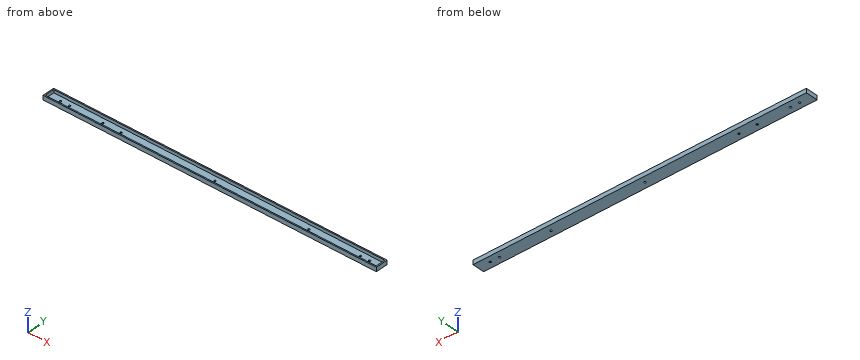
from build123d import *

# Parameters (mm, degrees)
SKETCH_1_W          = 550
SKETCH_1_H          = 20
EXTRUDE_1_DEPTH     = 7
SKETCH_2_W          = 546
SKETCH_2_H          = 16
CUT_EXTRUDE_1_DEPTH = 5
SKETCH_3_R          = 1.6
CUT_EXTRUDE_2_DEPTH = 276.270775783
SKETCH_4_R          = 1.6
CUT_EXTRUDE_3_DEPTH = 276.270775783


with BuildPart() as part:
    # ｽｹｯﾁ1 → ﾎﾞｽ - 押し出し1 (new body)
    with BuildSketch(Plane.XY):
        Rectangle(SKETCH_1_W, SKETCH_1_H)
    extrude(amount=EXTRUDE_1_DEPTH)

    # ｽｹｯﾁ2 → ｶｯﾄ - 押し出し1 (cut)
    with BuildSketch(Plane.XY.offset(7)):
        Rectangle(SKETCH_2_W, SKETCH_2_H)
    extrude(amount=-CUT_EXTRUDE_1_DEPTH, mode=Mode.SUBTRACT)

    # ｽｹｯﾁ3 → ｶｯﾄ - 押し出し2 (cut, through all)
    with BuildSketch(Plane(origin=(0, 0, 0), x_dir=(-1, 0, 0), z_dir=(0, 0, -1))):
        with Locations((255, 0)):
            Circle(SKETCH_3_R)
        with Locations((240, 0)):
            Circle(SKETCH_3_R)
        with Locations((155, 0)):
            Circle(SKETCH_3_R)
        Circle(SKETCH_3_R)
        with Locations(Location((-255, 0, 0), (0, 0, 180))):
            Circle(SKETCH_3_R)
        with Locations(Location((-240, 0, 0), (0, 0, 180))):
            Circle(SKETCH_3_R)
        with Locations(Location((-155, 0, 0), (0, 0, 180))):
            Circle(SKETCH_3_R)
    extrude(amount=-CUT_EXTRUDE_2_DEPTH, mode=Mode.SUBTRACT)

    # ｽｹｯﾁ4 → ｶｯﾄ - 押し出し3 (cut, through all)
    with BuildSketch(Plane(origin=(0, 0, 0), x_dir=(-1, 0, 0), z_dir=(0, 0, -1))):
        with Locations((185, 0)):
            Circle(SKETCH_4_R)
    extrude(amount=-CUT_EXTRUDE_3_DEPTH, mode=Mode.SUBTRACT)


solid = part.part
The model under review builds one solid part; all positions refer to its coordinate system, in mm. Coordinates: 2 decimals unless noted, no trailing zeros. Loops run counter-clockwise (first coordinate to the right, second up) from the corner with the lowest first, then second, coordinate; pieces in that order, holes last. Notation, with made-up numbers: (17, 76.25) -> (64, 76.25) arc R22 ccw to (64, 108.25) -> close; hole circle Ø4 at (-35.75, 0). An arc over 180 degrees is marked (long way). Use a Markdown table: item, result. Add a question column.
1. Clearance check with flat-ended pins moving along their axes: pin 1 Ø3.5 at (x, y) = (-155, 0) entering from -Z; pin 2 Ø3 at (x, y) = (255, 0) entering from -Z; pin 3 Ø5 at (x, y) = (68.5, 0.5) entering from +Z. State where each tip first meets the part, or that it passes through.
2. Add section A-A on z = 3.75. Write out the cut boundary in (x, y), plus the area to 3 significant figures.
3. To check wall thickness, follow line 1 (X direction, y = -2.5, z = 6); line 2 (Y direction, x = 7, z = 4.5); line 3 (Y direction, x = 0, z = 0.8). State the ranges of each line that lie inside material, in increasing order.
4. Add section B-B on x = 114.5. Write out the cut boundary in (y, z), plus the area to 3 significant figures.
Returned:
| question | item | result |
|---|---|---|
| 1 | pin 1 | stops at z = 0 |
| 1 | pin 2 | passes through |
| 1 | pin 3 | stops at z = 2 |
| 2 | outline | (-275, -10) -> (275, -10) -> (275, 10) -> (-275, 10) -> close; hole (-273, -8) -> (273, -8) -> (273, 8) -> (-273, 8) -> close |
| 2 | area | 2,260 mm² |
| 3 | line 1 | x = -275 to -273, 273 to 275 |
| 3 | line 2 | y = -10 to -8, 8 to 10 |
| 3 | line 3 | y = -10 to -1.6, 1.6 to 10 |
| 4 | outline | (-10, 0) -> (10, 0) -> (10, 7) -> (8, 7) -> (8, 2) -> (-8, 2) -> (-8, 7) -> (-10, 7) -> close |
| 4 | area | 60.0 mm² |
